```python
from build123d import *

# Parameters (mm, degrees)
F0_W      = 80
F0_H      = 50
F1_DEPTH  = 80
F1_FACE_W = 80
F1_FACE_H = 50
F2_DEPTH  = 80
F4_DEPTH  = 50


with BuildPart() as f1:
    # F0 (on Right) → F1 (new body)
    with BuildSketch(Plane.YZ):
        Rectangle(F0_W, F0_H)
    extrude(amount=F1_DEPTH)

    # F1_face (on face) → F2 (join)
    with BuildSketch(Plane(origin=(0, 0, 0), x_dir=(0, 1, 0), z_dir=(-1, 0, 0))):
        Rectangle(F1_FACE_W, F1_FACE_H)
    extrude(amount=F2_DEPTH)

    # F3 (on face) → F4 (cut)
    with BuildSketch(Plane.XY.offset(25)):
        with BuildLine():
            Line((80, -40), (80, 40))
            ThreePointArc((80, 40), (40, 0), (80, -40))
        make_face()
    extrude(amount=-F4_DEPTH, mode=Mode.SUBTRACT)


solid = f1.part
```
Work out the finished part from the listing and answer in its coordinate system (mm). Coordinates: 2 decimals unless noted, no trailing zeros. Loops run counter-clockwise (first coordinate to the right, second up) from the corner with the lowest first, then second, coordinate; pieces in that order, holes last. Notation, with made-up numbers: (5.5, 70.5) - (64.5, 70.5) arc R25 ccw to (64.5, 94.5) - close; hole circle Ø1 at (-29, -19). An arc over 180 degrees is marked (long way). Use a Markdown table: item, result.
Item 1: Given pin 1 Ø12 at (y, z) = (-19.5, 6) entering from +X; pin 2 Ø1.5 at (y, z) = (-27.5, 17.5) entering from +X, each flat-ended and moving along its own axis, determine where each tip first touches the part or whether it passes through.
Evaluation:
| item | result |
|---|---|
| pin 1 | stops at x = 49.18 |
| pin 2 | stops at x = 51.68 |
Item 2: Find section A-A, the plane x = 62. Determine the outline of the cut face in (y, z).
Evaluation:
| item | result |
|---|---|
| outline | (-40, -25) - (-35.72, -25) - (-35.72, 25) - (-40, 25) - close; (35.72, -25) - (40, -25) - (40, 25) - (35.72, 25) - close |
Item 3: Consider probe 1 along Y at (x, z) = (61, -8); probe 2 along Y at (x, z) = (47.5, -10.5); probe 3 along X at (y, z) = (1, -12). Determine where each line is inside the solid, lowest interval first. Write a range as from..to.
Evaluation:
| item | result |
|---|---|
| probe 1 | y = -40..-35.2, 35.2..40 |
| probe 2 | y = -40..-23.32, 23.32..40 |
| probe 3 | x = -80..40.01 |
Item 4: The mould has two halves that part along Y. Classify faces 1 (the flat face through (-80, -1, 0)), 2 (the flat face through (1, 40, 0)), 3 (the cylindrical face through (40.01, 0.88, 0.35)), 4 (the flat face through (1, -40, 0)): +Y half, -Y half, draft (parallel to the pull), parting line (faces both ways), or undercut.
Evaluation:
| item | result |
|---|---|
| face 1 | draft |
| face 2 | +Y half |
| face 3 | undercut |
| face 4 | -Y half |
Item 5: Find section C-C, the plane y = 0. Determine the outline of the cut face in (x, z).
Evaluation:
| item | result |
|---|---|
| outline | (-80, -25) - (40, -25) - (40, 25) - (-80, 25) - close |
Item 6: Find section B-B, the plane z = -5. Determine the outline of the cut face in (x, y), and give its area (3 significant figures).
Evaluation:
| item | result |
|---|---|
| outline | (-80, -40) - (80, -40) arc R40 cw to (80, 40) - (-80, 40) - close |
| area | 10,300 mm2 |
